Can you work these out from the model? Positions are in its coordinate system, mm. Face numbers are marked on the shaded views. A direction names the side the tool comes from. Give positions to 0.01 mm unless a question says otherwise; leave off trailing zeros. Loops run counter-clockwise (first coordinate to the right, second up) from the corner with the lowest first, then second, coordinate; pieces in that order, holes last. Notation, with made-up numbers: (-10.5, -21) -> (39.5, -21) arc R15 cw to (39.5, 1) -> close; hole circle Ø9 at (7, 4.5). An arc over 180 degrees is marked (long way). Return JSON: item names as keys, results as strings. Group by question number.
Q1. Which directions (+Z, -Z, +X, -X, +Y, -Y) give clear straight access to the entire face, cutting with the end or side of a thin tool? Please do the marked faces 4, 5 and 6.
Q2. Thinking about a two-plate mould opening in X: for the marked faces 1, 2 and 3, which applies, pulls with the +X half, pulls with the -X half, needs draft (parallel to the pull), parting line crosses it, or undercut?
Q3. Will these pins go through, and if not, where does the flat tip stop? pin 1 (3.5 mm diameter, centred on x = -3, z = 3.5, fed in from -Y); pin 2 (1.1 mm diameter, centred on y = -4.5, z = 6.5, fed in from -X).
Q4. Suppose I cut it at C-C, the plane y = -11. Please give me the cut outline in (x, z), and give its area (3 significant figures).
Q5. I need wall thicknesses on line 1 along Z through (x, y) = (1.5, -11); line 2 along Y through (x, z) = (2.45, 3.5); line 3 along Y through (x, z) = (-1, -2). Which ranges of each line are inside material? Lowest first, please. Write a range as [from, to].
Q6. Suppose I cut it at B-B, the plane z = 3.5. Please give me the cut outline in (x, y).
Q7. Suppose I cut it at D-D, the plane y = -2.75. Please give me the cut outline in (x, z).
Q8. Suppose I cut it at A-A, the plane x = -3. Please give me the cut outline in (y, z), and give its area (3 significant figures).
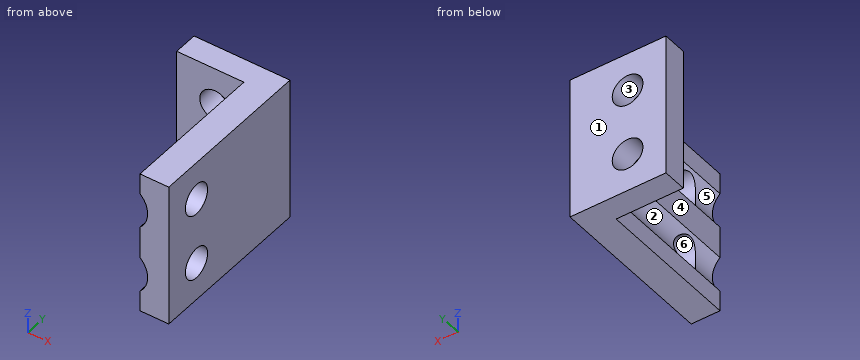
```python
from build123d import *

# Parameters (mm, degrees)
BOSS_EXTRUDE1_DEPTH = 7.5
SKETCH2_R           = 1.6
CUT_EXTRUDE1_DEPTH  = 15
SKETCH3_R           = 1.6
CUT_EXTRUDE2_DEPTH  = 15
SKETCH4_R           = 2.5
CUT_EXTRUDE3_DEPTH  = 15


with BuildPart() as part:
    # Sketch1 → Boss-Extrude1 (new, symmetric)
    with BuildSketch(Plane.XY):
        Polygon((0, 0), (-7, 0), (-7, 2.5), (3, 2.5), (3, -15), (0, -15), align=None)
    extrude(amount=BOSS_EXTRUDE1_DEPTH, both=True)

    # Sketch2 → Cut-Extrude1 (cut)
    with BuildSketch(Plane(origin=(0, 2.5, 0), x_dir=(1, 0, 0), z_dir=(0, 1, 0))):
        with Locations(Location((-3, 3.5, 0), (0, 0, 270))):
            Circle(SKETCH2_R)
        with Locations(Location((-3, -3.5, 0), (0, 0, 270))):
            Circle(SKETCH2_R)
    extrude(amount=-CUT_EXTRUDE1_DEPTH, mode=Mode.SUBTRACT)

    # Sketch3 → Cut-Extrude2 (cut)
    with BuildSketch(Plane(origin=(3, 0, 0), x_dir=(0, 0, -1), z_dir=(1, 0, 0))):
        with Locations(Location((3.5, -11, 0), (0, 0, 90))):
            Circle(SKETCH3_R)
        with Locations(Location((-3.5, -11, 0), (0, 0, 90))):
            Circle(SKETCH3_R)
    extrude(amount=-CUT_EXTRUDE2_DEPTH, mode=Mode.SUBTRACT)

    # Sketch4 → Cut-Extrude3 (cut)
    with BuildSketch(Plane.XZ.offset(15)):
        with Locations((-1.7, 3.5)):
            Circle(SKETCH4_R)
        with Locations((-1.7, -3.5)):
            Circle(SKETCH4_R)
    extrude(amount=-CUT_EXTRUDE3_DEPTH, mode=Mode.SUBTRACT)


solid = part.part
```
Ans:
{
 "1": {"face 4": "+Z, -Z, -X, -Y", "face 5": "-X, -Y", "face 6": "+X, -X"},
 "2": {"face 1": "needs draft", "face 2": "pulls with the -X half", "face 3": "undercut"},
 "3": {"pin 1": "stops at y = 0", "pin 2": "stops at x = 0"},
 "4": {"outline": "(0, -7.5) -> (3, -7.5) -> (3, -5.1) -> (0.22, -5.1) arc R2.5 cw to (0, -5.33) -> close; (0, -1.67) arc R2.5 cw to (0.22, -1.9) -> (3, -1.9) -> (3, 1.9) -> (0.22, 1.9) arc R2.5 cw to (0, 1.67) -> close; (0, 5.33) arc R2.5 cw to (0.22, 5.1) -> (3, 5.1) -> (3, 7.5) -> (0, 7.5) -> close", "area": "25.7 mm^2"},
 "5": {"line 1": "z = [-7.5, -5.1], [-1.9, 1.9], [5.1, 7.5]", "line 2": "y = [-15, -12.6], [-9.4, 2.5]", "line 3": "y = [0, 2.5]"},
 "6": {"outline": "(-7, 0) -> (-4.6, 0) -> (-4.6, 2.5) -> (-7, 2.5) -> close; (-1.4, 0) -> (0.8, 0) -> (0.8, -9.4) -> (3, -9.4) -> (3, 2.5) -> (-1.4, 2.5) -> close; (0.8, -15) -> (3, -15) -> (3, -12.6) -> (0.8, -12.6) -> close"},
 "7": {"outline": "(0, -7.5) -> (3, -7.5) -> (3, 7.5) -> (0, 7.5) -> (0, 5.33) arc R2.5 cw to (0, 1.67) -> (0, -1.67) arc R2.5 cw to (0, -5.33) -> close"},
 "8": {"outline": "(0, -7.5) -> (2.5, -7.5) -> (2.5, -5.1) -> (0, -5.1) -> close; (0, -1.9) -> (2.5, -1.9) -> (2.5, 1.9) -> (0, 1.9) -> close; (0, 5.1) -> (2.5, 5.1) -> (2.5, 7.5) -> (0, 7.5) -> close", "area": "21.5 mm^2"}
}
